Drawing for the job (mm, zero at the part's lowest x, y, z). A direction names the side the tool comes from. Give positions to 0.01 mm unless a question says otherwise; leave off trailing zeros. Loops run counter-clockwise (first coordinate to the right, second up) from the corner with the lowest first, then second, coordinate; pieces in that order, holes last.
1) Two-plate mould, pull along Y, no slides. Class the marked faces 6, 7 and 8: +Y half, -Y half, draft (parallel to the pull), parting line (faces both ways), or undercut.
2) Band-saw the part on D-D on z = 5. List the corners of the cut face in (x, y), then the cut area to 3 significant figures.
3) Wall check: line 1 (X direction, y = 4.55, z = 3.55); line 2 (Z direction, x = 4.2, y = 3); line 3 (Y direction, x = 3.6, z = 2.15). Give the ranges that are in metal, low to high.
4) Flat gauge pins, fed straight in: P1, Ø1.5, axis at y = 4, z = 2.5, coming from the +X side; P2, Ø1.1, axis at x = 2, z = 2, coming from the +Y side; P3, Ø2.5, axis at y = 3.5, z = 2.5, coming from the -X side. Where does each tip first touch, or does it go through?
5) Band-saw the part on A-A on z = 2.9. List the corners of the cut face in (x, y), then the cut area to 3 significant figures.
6) Band-saw the part on C-C on y = 2.8. List the corners of the cut face in (x, z).
7) 3-axis set-ups, long thin cutter, end or side, ignore diameter. For the marked faces 1, 2, 3, 4 and 5: which of +Z, -Z, +X, -X, +Y, -Y reach the whole face in a straight line?
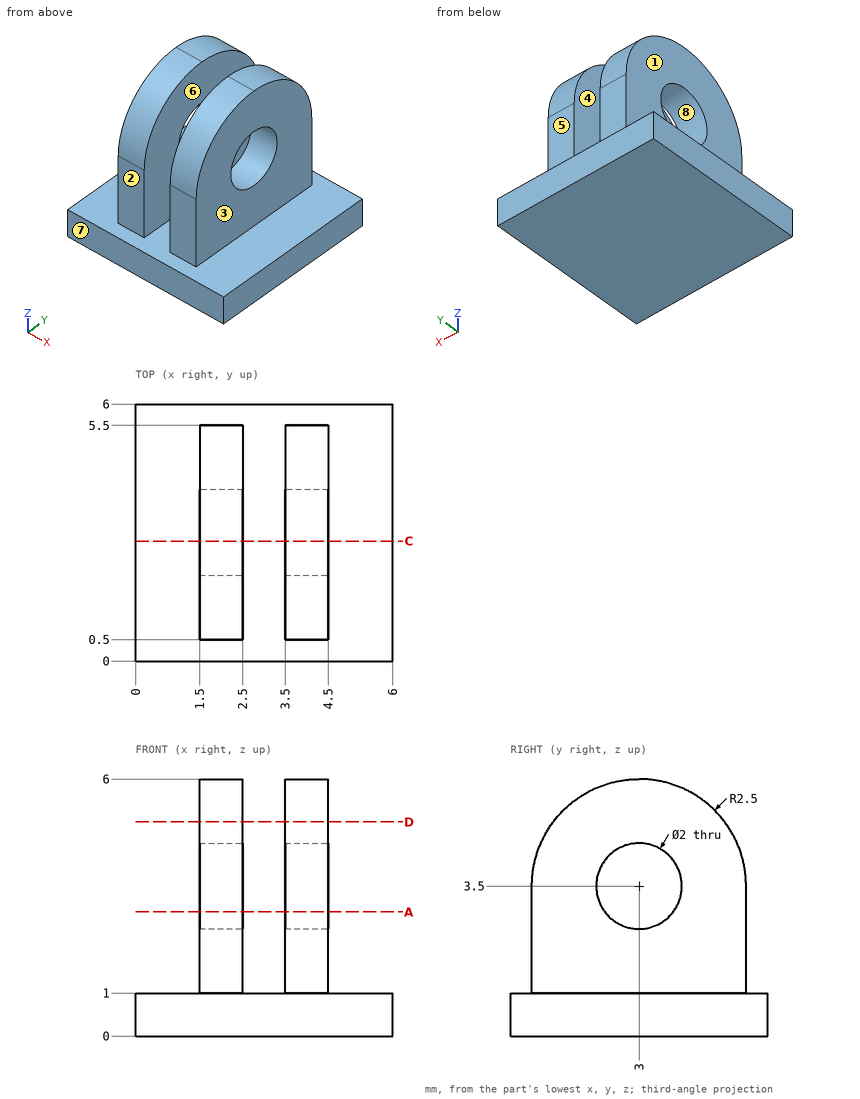
Findings below:
1. face 6: draft
1. face 7: -Y half
1. face 8: undercut
2. outline: (1.5, 1) - (2.5, 1) - (2.5, 5) - (1.5, 5) - close; (3.5, 1) - (4.5, 1) - (4.5, 5) - (3.5, 5) - close
2. area: 8.00 mm2
3. line 1: x = 1.5 to 2.5, 3.5 to 4.5
3. line 2: z = 0 to 2.5, 4.5 to 6
3. line 3: y = 0.5 to 5.5
4. P1: stops at x = 4.5
4. P2: stops at y = 5.5
4. P3: stops at x = 1.5
5. outline: (1.5, 0.5) - (2.5, 0.5) - (2.5, 2.2) - (1.5, 2.2) - close; (1.5, 3.8) - (2.5, 3.8) - (2.5, 5.5) - (1.5, 5.5) - close; (3.5, 0.5) - (4.5, 0.5) - (4.5, 2.2) - (3.5, 2.2) - close; (3.5, 3.8) - (4.5, 3.8) - (4.5, 5.5) - (3.5, 5.5) - close
5. area: 6.80 mm2
6. outline: (0, 0) - (6, 0) - (6, 1) - (4.5, 1) - (4.5, 2.52) - (3.5, 2.52) - (3.5, 1) - (2.5, 1) - (2.5, 2.52) - (1.5, 2.52) - (1.5, 1) - (0, 1) - close; (1.5, 4.48) - (2.5, 4.48) - (2.5, 5.99) - (1.5, 5.99) - close; (3.5, 4.48) - (4.5, 4.48) - (4.5, 5.99) - (3.5, 5.99) - close
7. face 1: +Z, -X, +Y, -Y
7. face 2: +Z, +X, -X, -Y
7. face 3: +Z, +X, +Y, -Y
7. face 4: +Z, +Y, -Y
7. face 5: +Z, +X, -X, +Y
